Could you check a few things on this drawing? It's one solid part, dimensions in mm from its lowest x, y, z. A direction names the side the tool comes from. Coordinates: 2 decimals unless noted, no trailing zeros. Write each loop counter-clockwise with the first axis right and the second up, starting at its lowest first coordinate (ties: lowest second). Pieces come first, ordered by that corner, then holes. Notation, with made-up numbers: (63, -2.75) - (72, -2.75) arc R25 ccw to (72, 25.25) - close; hole circle Ø9 at (55.25, -9.75). An arc over 180 degrees is marked (long way). Use one line per item in the form item = value. Start each with the question number.
(1) For pin 1 Ø9 at (x, y) = (75, 22.5) entering from -Z; pin 2 Ø4 at (y, z) = (19.5, 3) entering from -X; pin 3 Ø1 at (x, y) = (50.5, 39) entering from +Z; pin 4 Ø22.5 at (x, z) = (34.5, 17.5) entering from -Y, each with a flat end and sliding along its axis, tell me the tip position at first contact or that it passes through.
(2) On a 3-axis mill with a long thin cutter (end or side, diameter ignored), from which of +Z, -Z, +X, -X, +Y, -Y can I reach the whole of each face in a straight line? I mean the marked faces 1, 2, 3, 4 and 5. Say none if no direction works.
(3) If we section it at C-C on x = 75: Please give me the cut outline in (y, z), then the cut area to 3 significant figures.
(4) If we section it at A-A on z = 32: Please give me the cut outline in (x, y), then the cut area to 3 significant figures.
(5) If I drill on probe 1 along Z at (x, y) = (67, 2.5); probe 2 along Y at (x, z) = (45.5, 4.5); probe 3 along Y at (x, z) = (75, 39.25), over which ranges is the centre line in solid material (lowest first)? Write a range as from..to.
(6) Thinking about a two-plate mould opening in X: for the marked faces 6, 7 and 8, which applies, pulls with the +X half, pulls with the -X half, needs draft (parallel to the pull), parting line crosses it, or undercut?
(7) If we section it at D-D on y = 22.5: Please give me the cut outline in (x, z).
(8) If we section it at B-B on y = 31.5: Please give me the cut outline in (x, z).
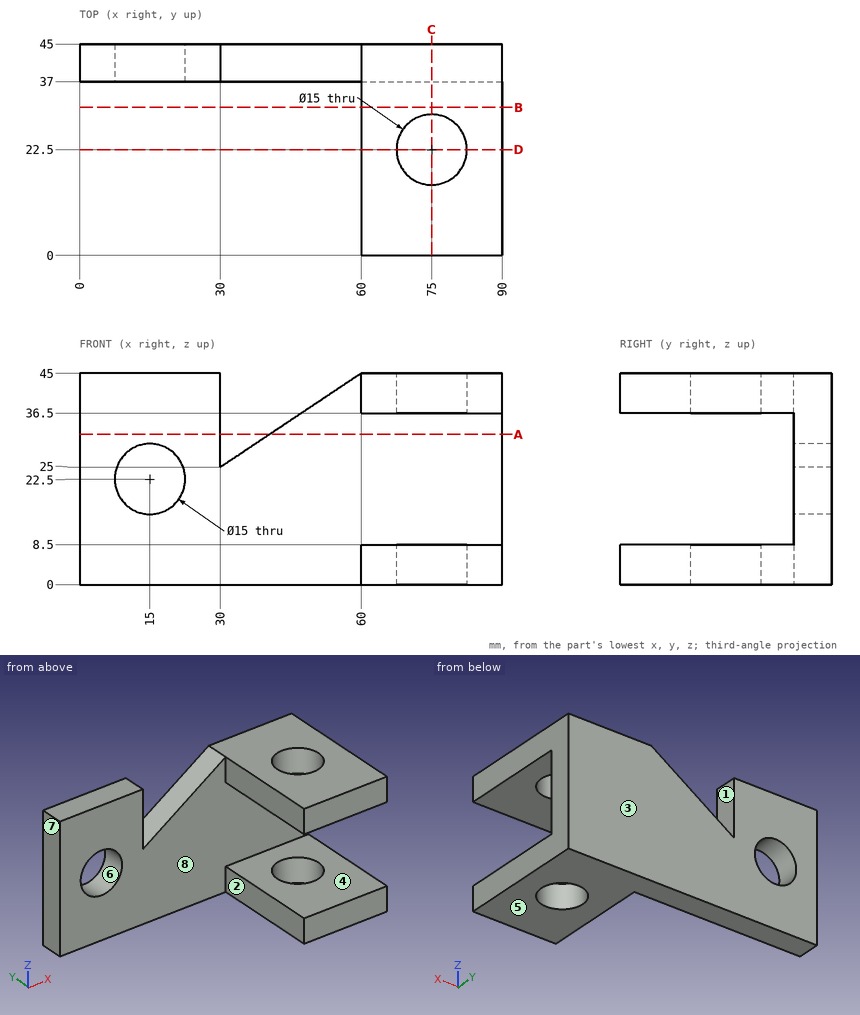
Reported:
q1.pin_1 = through
q1.pin_2 = 60
q1.pin_3 = 39
q1.pin_4 = 37
q2.face_1 = +Z, +Y, -Y
q2.face_2 = +Z, -Z, -X, -Y
q2.face_3 = +Z, -Z, +X, -X, +Y
q2.face_4 = +X, -X, -Y
q2.face_5 = -Z, +X, -X, +Y, -Y
q3.outline = (0, 0) - (15, 0) - (15, 8.5) - (0, 8.5) - close; (0, 36.5) - (15, 36.5) - (15, 45) - (0, 45) - close; (30, 0) - (45, 0) - (45, 45) - (30, 45) - (30, 36.5) - (37, 36.5) - (37, 8.5) - (30, 8.5) - close
q3.area = 734 mm2
q4.outline = (0, 37) - (30, 37) - (30, 45) - (0, 45) - close; (40.5, 37) - (90, 37) - (90, 45) - (40.5, 45) - close
q4.area = 636 mm2
q5.probe_1 = 0..8.5, 36.5..45
q5.probe_2 = 37..45
q5.probe_3 = 0..15, 30..45
q6.face_6 = undercut
q6.face_7 = pulls with the -X half
q6.face_8 = needs draft
q7.outline = (60, 0) - (67.5, 0) - (67.5, 8.5) - (60, 8.5) - close; (60, 36.5) - (67.5, 36.5) - (67.5, 45) - (60, 45) - close; (82.5, 0) - (90, 0) - (90, 8.5) - (82.5, 8.5) - close; (82.5, 36.5) - (90, 36.5) - (90, 45) - (82.5, 45) - close
q8.outline = (60, 0) - (90, 0) - (90, 8.5) - (60, 8.5) - close; (60, 36.5) - (90, 36.5) - (90, 45) - (60, 45) - close
